For this review, take the finished solid that the model builds, in its own axes (mm). A direction names the side the tool comes from. Give positions to 0.01 mm unless a question says otherwise; leave off trailing zeros. Loops run counter-clockwise (first coordinate to the right, second up) from the corner with the lowest first, then second, coordinate; pieces in that order, holes last.
Autodesk Inventor part; units mm, degrees
ref_plane "YZ Plane" through (0, 0, 0) normal (1, 0, 0) x (0, 1, 0)
ref_plane "XZ Plane" through (0, 0, 0) normal (0, 1, 0) x (-1, 0, 0)
ref_plane "XY Plane" through (0, 0, 0) normal (0, 0, 1) x (1, 0, 0)
sketch "Sketch1" plane through (0, 0, 0) normal (0, 0, 1) x (1, 0, 0)
  line L0 (-25.5, -25.5) -> (25.5, -25.5)
  line L1 (25.5, -25.5) -> (25.5, 25.5)
  line L2 (25.5, 25.5) -> (-25.5, 25.5)
  line L3 (-25.5, 25.5) -> (-25.5, -25.5)
  line L4 (-25.5, -25.5) -> (25.5, 25.5) construction
  line L5 (25.5, -25.5) -> (-25.5, 25.5) construction
  point P0 (0, 0)
  dimension "d0" = 51
  dimension "d1" = 51
extrude "Extrusion1" add sketch "Sketch1" against normal blind 2.921
sketch "Sketch4" plane through (0, 0, 0) normal (0, 0, 1) x (1, 0, 0)
  line L0 (-25.5, -25.5) -> (-9.5, -25.5)
  line L1 (-9.5, -25.5) -> (-9.5, -22.5)
  line L2 (-9.5, -22.5) -> (-25.5, -22.5)
  line L3 (-25.5, -22.5) -> (-25.5, -25.5)
  line L4 (25.5, 25.5) -> (-25.5, 25.5)
  line L5 (-25.5, 25.5) -> (-25.5, -25.5)
  line L6 (-25.5, 18.5) -> (-22.5, 18.5)
  line L7 (-22.5, 18.5) -> (-22.5, -0.5)
  line L8 (-22.5, -0.5) -> (-25.5, -0.5)
  line L9 (-25.5, -0.5) -> (-25.5, 18.5)
  line L10 (25.5, -0.5) -> (25.5, 18.5)
  line L11 (-9.5, 25.5) -> (9.5, 25.5)
  line L12 (9.5, 25.5) -> (9.5, 22.5)
  line L13 (9.5, 22.5) -> (-9.5, 22.5)
  line L14 (-9.5, 22.5) -> (-9.5, 25.5)
  line L15 (-25.5, -25.5) -> (25.5, -25.5)
  line L16 (25.5, -25.5) -> (25.5, 25.5)
  line L17 (25.5, -0.5) -> (22.5, -0.5)
  line L18 (22.5, -0.5) -> (22.5, -22.5)
  line L19 (22.5, -25.5) -> (25.5, -25.5)
  line L20 (25.5, -25.5) -> (25.5, -0.5)
  line L21 (25.5, -25.5) -> (9.5, -25.5)
  line L22 (9.5, -25.5) -> (9.5, -22.5)
  line L23 (9.5, -22.5) -> (22.5, -22.5)
  line L24 (25.5, -22.5) -> (25.5, -25.5)
  line L25 (25.5, 25.5) -> (22.5, 25.5)
  line L26 (22.5, 25.5) -> (22.5, 18.5)
  line L27 (22.5, 18.5) -> (25.5, 18.5)
  line L28 (25.5, 18.5) -> (25.5, 25.5)
  point P0 (0, 0)
  dimension "d16" = 3
  dimension "d37" = 9.5
  dimension "d38" = 16
  dimension "d40" = 3
  dimension "d42" = 19
  dimension "d44" = 3
  dimension "d45" = 19
  dimension "d46" = 16
  dimension "d50" = 25
  dimension "d62" = 3
  dimension "d63" = 25
  dimension "d64" = 3
  dimension "d65" = 19
  dimension "d66" = 16
  dimension "d67" = 3
  dimension "d68" = 7
  dimension "d71" = 19
  dimension "d72" = 7
hole "Hole1" at (-0.1, 0, 0) direction (0, 0, -1) diameter 25.4 end through all
extrude "Extrusion6" cut sketch "Sketch4" against normal up to next contours L3 L2 L1 L0 | L22 L23 L18 L17 L16 L15 | L5 L6 L7 L8 | L4 L12 L13 L14 | L27 L26 L4 L16
equation "\"d1\" = d0"
equation "\"d16\" = d44"
equation "\"d38\" = -d37 + 0.5 * d0"
equation "\"d40\" = d44"
equation "\"d42\" = d45"
equation "\"d46\" = -0.5 * d45 + 0.5 * d52"
equation "\"d62\" = d44"
equation "\"d63\" = d50"
equation "\"d64\" = d44"
equation "\"d65\" = d45"
equation "\"d67\" = d44"
equation "\"d71\" = d42"
equation "\"d48\" = 0.5 * d0"
properties part number "Side B"
Item 1: Tool access review of faces 1 (the flat face through (22.5, 22, -1)), 2 (the flat face through (-24, 18.5, -1)), 3 (the flat face through (-17, -22.5, -1)), 4 (the flat face through (24, -0.5, -1)): name each direction out of +Z, -Z, +X, -X, +Y, -Y from which nothing blocks a thin tool from reaching the whole face with its end or side.
Answer:
face 1: +Z, -Z, +X, +Y
face 2: +Z, -Z, -X
face 3: +Z, -Z, -X, -Y
face 4: +Z, -Z, +X, -Y
Item 2: Clearance check with flat-ended pins moving along their axes: pin 1 Ø0.9 at (y, z) = (-23.5, -2) entering from +X; pin 2 Ø1.5 at (x, z) = (23.5, -2) entering from -Y; pin 3 Ø10 at (x, y) = (-4, 0.5) entering from -Z; pin 4 Ø1.5 at (x, z) = (-16, -1.5) entering from -Y. State where each tip first meets the part, or that it passes through.
Answer:
pin 1: stops at x = 9.5
pin 2: stops at y = -0.5
pin 3: passes through
pin 4: stops at y = -22.5
Item 3: The part is to be moulded in two halves that separate along X. For faces 5 (the flat face through (9.5, 24, -1)), 6 (the flat face through (0, 22.5, -1)), 7 (the flat face through (16, 25.5, -1)), 8 (the flat face through (-25.5, 22, -1)), say which applies: released by +X, released by -X, zero draft, split by the parting line, or undercut.
Answer:
face 5: undercut
face 6: undercut
face 7: zero draft
face 8: released by -X
Item 4: Take a section at D-D on y = -13.5. Give the boundary of the cut face in (x, z).
Answer:
outline: (-25.5, -2.92) - (22.5, -2.92) - (22.5, 0) - (-25.5, 0) - close
Item 5: Take a section at B-B on y = -6. Give the boundary of the cut face in (x, z), and give its area (3 significant figures).
Answer:
outline: (-25.5, -2.92) - (-11.29, -2.92) - (-11.29, 0) - (-25.5, 0) - close; (11.09, -2.92) - (22.5, -2.92) - (22.5, 0) - (11.09, 0) - close
area: 74.8 mm2
Item 6: Take a section at A-A on x = -0.1. Give the boundary of the cut face in (y, z).
Answer:
outline: (-25.5, -2.92) - (-12.7, -2.92) - (-12.7, 0) - (-25.5, 0) - close; (12.7, -2.92) - (22.5, -2.92) - (22.5, 0) - (12.7, 0) - close
Item 7: For L1, parallel to X at y = 0, z = -1.3; L2, parallel to Y at x = -0.1, z = -1.4; L3, parallel to X at y = -15, z = -2.15, list the stretches that pass through material, from the lowest coordinate up.
Answer:
L1: x = -22.5 to -12.8, 12.6 to 25.5
L2: y = -25.5 to -12.7, 12.7 to 22.5
L3: x = -25.5 to 22.5
Item 8: Take a section at C-C on z = -1.25. Give the boundary of the cut face in (x, y), and give its area (3 significant figures).
Answer:
outline: (-25.5, -22.5) - (-9.5, -22.5) - (-9.5, -25.5) - (9.5, -25.5) - (9.5, -22.5) - (22.5, -22.5) - (22.5, -0.5) - (25.5, -0.5) - (25.5, 18.5) - (22.5, 18.5) - (22.5, 25.5) - (9.5, 25.5) - (9.5, 22.5) - (-9.5, 22.5) - (-9.5, 25.5) - (-25.5, 25.5) - (-25.5, 18.5) - (-22.5, 18.5) - (-22.5, -0.5) - (-25.5, -0.5) - close; hole circle Ø25.4 at (-0.1, 0)
area: 1,800 mm2
